```python
from build123d import *

# Parameters (mm, degrees)
SKETCH1_W                      = 50
SKETCH1_H                      = 50
BOSS_EXTRUDE1_DEPTH            = 45
SKETCH3_R                      = 11
BOSS_EXTRUDE2_DEPTH            = 37
BOSS_EXTRUDE3_DEPTH            = 6
SKETCH5_W                      = 34
SKETCH5_H                      = 34
CUT_EXTRUDE1_DEPTH             = 103.127371453
F_12_5_12_5_DIAMETER_HOLE1_D   = 12.5
F_12_0_START                   = 17
F_12_0_12_DIAMETER_SLOT2_DEPTH = 14
F_10_0_START                   = 17
F_10_0_10_DIAMETER_SLOT1_DEPTH = 8
M10_CLEARANCE_HOLE1_D          = 11
M10_CLEARANCE_HOLE1_DEPTH      = 8
M10_CLEARANCE_HOLE2_D          = 11
M10X1_0_TAPPED_HOLE1_D         = 9
M10X1_0_TAPPED_HOLE1_DEPTH     = 8


# Read off the part's stored shape, not the designer's step: Ø12.0 (12) Diameter Slot2, Ø10.0 (10) Diameter Slot1
with BuildPart() as part:
    # Sketch1 → Boss-Extrude1 (new, symmetric)
    with BuildSketch(Plane(origin=(0, 0, 0), x_dir=(0, 0, -1), z_dir=(1, 0, 0))):
        Rectangle(SKETCH1_W, SKETCH1_H)
    extrude(amount=BOSS_EXTRUDE1_DEPTH, both=True)

    # Sketch3 → Boss-Extrude2 (add, symmetric)
    with BuildSketch(Plane.XY):
        Circle(SKETCH3_R)
    extrude(amount=BOSS_EXTRUDE2_DEPTH, both=True)

    # Sketch4 → Boss-Extrude3 (add)
    with BuildSketch(Plane(origin=(0, 25, 0), x_dir=(1, 0, 0), z_dir=(0, 1, 0))):
        with BuildLine():
            Line((-10, 11), (10, 11))
            ThreePointArc((10, 11), (21, 0), (10, -11))
            Line((10, -11), (-10, -11))
            ThreePointArc((-10, -11), (-21, 0), (-10, 11))
        make_face()
    extrude(amount=BOSS_EXTRUDE3_DEPTH)

    # Sketch5 → Cut-Extrude1 (cut, through all)
    with BuildSketch(Plane(origin=(45, 0, 0), x_dir=(0, 0, -1), z_dir=(1, 0, 0))):
        Rectangle(SKETCH5_W, SKETCH5_H)
    extrude(amount=-CUT_EXTRUDE1_DEPTH, mode=Mode.SUBTRACT)

    # Ø12.5 (12.5) Diameter Hole1 (through all)
    with Locations(Plane.XY.offset(37)):
        with Locations((0, 0)):
            Hole(F_12_5_12_5_DIAMETER_HOLE1_D / 2)

    # Ø12.0 (12) Diameter Slot2 outline → Ø12.0 (12) Diameter Slot2 (cut)
    with BuildSketch(Plane(origin=(0, 0, 0), x_dir=(1, 0, 0), z_dir=(0, 1, 0)).offset(F_12_0_START)):
        with BuildLine():
            Line((-10, -6), (10, -6))
            ThreePointArc((10, -6), (16, 0), (10, 6))
            Line((10, 6), (-10, 6))
            ThreePointArc((-10, 6), (-16, 0), (-10, -6))
        make_face()
    extrude(amount=F_12_0_12_DIAMETER_SLOT2_DEPTH, mode=Mode.SUBTRACT)

    # Ø10.0 (10) Diameter Slot1 outline → Ø10.0 (10) Diameter Slot1 (cut)
    with BuildSketch(Plane(origin=(0, 0, 0), x_dir=(1, 0, 0), z_dir=(0, 1, 0)).offset(F_10_0_START)):
        with BuildLine():
            ThreePointArc((35, 12), (30, 7), (35, 2))
            Line((35, 2), (45, 2))
            Line((45, 2), (45, 12))
            Line((45, 12), (35, 12))
        make_face()
    extrude(amount=F_10_0_10_DIAMETER_SLOT1_DEPTH, mode=Mode.SUBTRACT)

    # M10 Clearance Hole1
    with Locations(Plane(origin=(0, 25, 0), x_dir=(1, 0, 0), z_dir=(0, 1, 0))):
        with Locations((-35, -7)):
            Hole(M10_CLEARANCE_HOLE1_D / 2, depth=M10_CLEARANCE_HOLE1_DEPTH)

    # M10 Clearance Hole2 (through all)
    with Locations(Plane(origin=(35, 0, 25), x_dir=(1, 0, 0), z_dir=(0, 0, 1))):
        with Locations((0, 0)):
            Hole(M10_CLEARANCE_HOLE2_D / 2)

    # M10x1.0 Tapped Hole1
    with Locations(Plane(origin=(0, 0, -25), x_dir=(-1, 0, 0), z_dir=(0, 0, -1))):
        with Locations((32.490263529, 0)):
            Hole(M10X1_0_TAPPED_HOLE1_D / 2, depth=M10X1_0_TAPPED_HOLE1_DEPTH)


solid = part.part
```
The listing builds one solid part. Answer for the finished solid, in the listing's coordinates (mm). A direction names the side the tool comes from. Give positions to 0.01 mm unless a question says otherwise; leave off trailing zeros. Order: outer loops, then holes, each group sorted by start corner. A loop starts at its lowest first (then second) coordinate and runs counter-clockwise, first axis right, second up.
Item 1: The part is cut by section D-D, the plane x = -35. Give the vertices of the cut face in (y, z), and give its area (3 significant figures).
From the geometry:
outline: (-25, -25) - (-3.74, -25) - (-3.74, -17) - (-17, -17) - (-17, 17) - (17, 17) - (17, 12.5) - (25, 12.5) - (25, 25) - (-25, 25) - close; (3.74, -25) - (25, -25) - (25, 1.5) - (17, 1.5) - (17, -17) - (3.74, -17) - close
area: 1,200 mm2
Item 2: The part is cut by section B-B, the plane z = 15. Give the vertices of the cut face in (x, y), and give its area (3 significant figures).
From the geometry:
outline: (-45, -25) - (45, -25) - (45, -17) - (-45, -17) - close; (-45, 17) - (45, 17) - (45, 25) - (-45, 25) - close
area: 1,440 mm2
Item 3: For a pull along Y with two mould halves and no side action, classify faces 1 (the face through (40.495, 0.242, 20.944)), 2 (the face through (0.6, -11.5, -25)), 3 (the face through (-2.38, -10.74, 31.08)) as pulls with the +Y half, pulls with the -Y half, needs draft (parallel to the pull), parting line crosses it, or undercut.
From the geometry:
face 1: undercut
face 2: needs draft
face 3: parting line crosses it
Item 4: Find the intervals of material crossed by probe 1 along Z at (x, y) = (-25, -6); probe 2 along Z at (x, y) = (-35, 19.25), in increasing order.
From the geometry:
probe 1: z = -25 to -17, 17 to 25
probe 2: z = -25 to 1.5, 12.5 to 25
Item 5: Which of the six approach directions +Z, -Z, +X, -X, +Y, -Y give full straight-line access (tool end or side, diameter ignored) to faces 4 (the face through (0.6, -11.5, 25)), 5 (the face through (-16, 24, 0)), 6 (the face through (-21, 28, 0)), 7 (the face through (1, 7, 17))?
From the geometry:
face 4: +Z
face 5: +Y
face 6: -X, +Y
face 7: +X, -X
Item 6: Given pin 1 Ø2.5 at (x, y) = (40, 22) entering from +Z; pin 2 Ø12 at (y, z) = (-7.5, 8) entering from +X; pin 3 Ø10.5 at (x, y) = (-32.49, 0) entering from -Z; pin 4 Ø3 at (x, y) = (1, 27) entering from +Z, each flat-ended and moving along its own axis, determine where each tip first touches the part or whether it passes through.
From the geometry:
pin 1: stops at z = 25
pin 2: passes through
pin 3: stops at z = -25
pin 4: stops at z = 11
Item 7: The part is cut by section A-A, the plane x = 0. Count the separate pieces of the cut face and the enclosed holes in it, and give its area (3 significant figures).
From the geometry:
separate pieces: 3
enclosed holes: 0
area: 1,340 mm2
